Verification items for this drawing (mm, ordinates from the low corner). Coordinates: 2 decimals unless noted, no trailing zeros. Order: outer loops, then holes, each group sorted by start corner. A loop starts at its lowest first (then second) coordinate and runs counter-clockwise, first axis right, second up. Notation, with made-up numbers: M 52.5,41.5 L 69.5,41.5 A26 cw 69.5,77.5 Z; hole C 9,4 d10. An arc over 180 degrees is marked long. Return JSON: item names as keys, results as strings. Group by question number.
1. Gauge pin test, flat ends, axial feed: pin 1 (0.5 mm diameter, centred on x = 6, y = 1, fed in from -Z); pin 2 (0.8 mm diameter, centred on y = 0.5, z = 21.5, fed in from -X); pin 3 (0.8 mm diameter, centred on y = 1, z = 22.5, fed in from +X). Record the tip position at first contact, or that the pin passes through.
2. Section check A-A, the plane y = 0.3. Record the cut outline in (x, z), plus the area to 3 significant figures.
3. Section check C-C, the plane x = 24. Record the cut outline in (y, z), plus the area to 3 significant figures.
4. Material ranges on line 1 along X through (y, z) = (0.7, 9); line 2 along X through (y, z) = (0.55, 23), recorded low to high.
5. Section check B-B, the plane z = 9.5. Record the cut outline in (x, y), plus the area to 3 significant figures.
6. Section check D-D, the plane z = 20. Record the cut outline in (x, y).
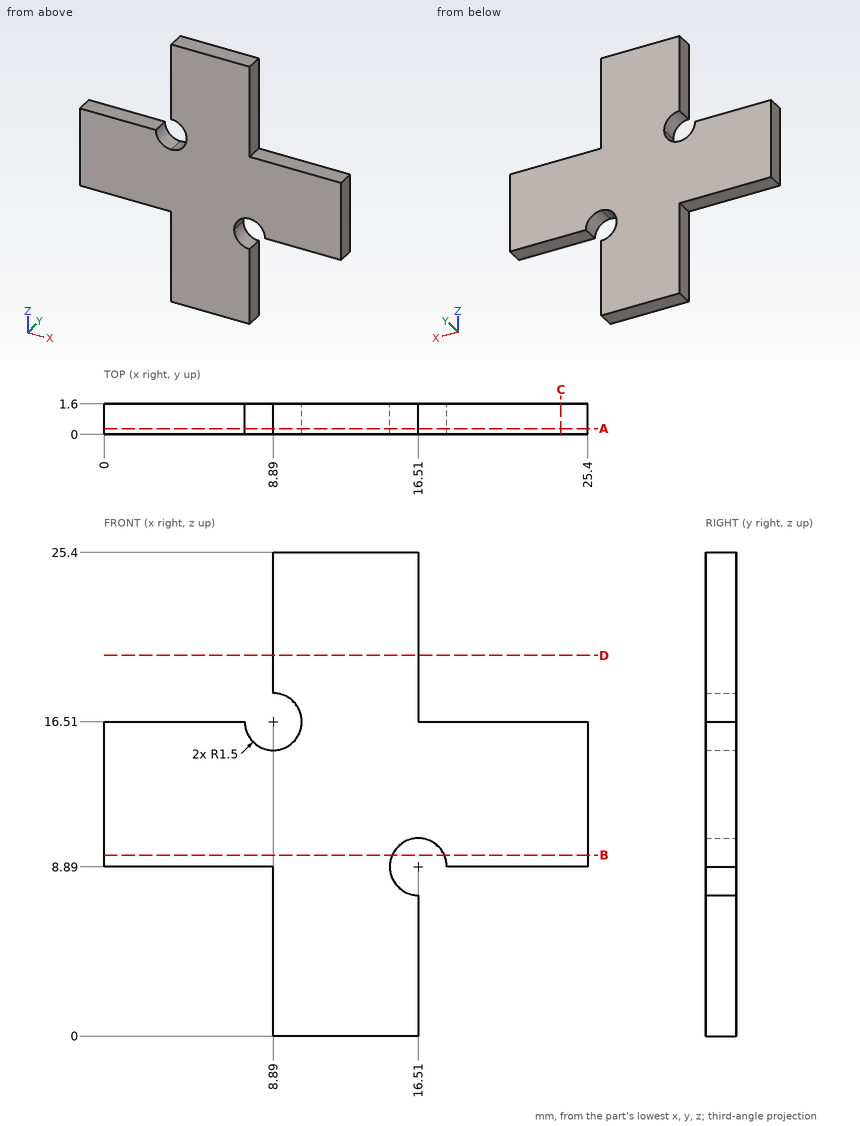
Answers follow:
{
 "1": {"pin 1": "z = 8.89", "pin 2": "x = 8.89", "pin 3": "x = 16.51"},
 "2": {"outline": "M 0,8.89 L 8.89,8.89 L 8.89,0 L 16.51,0 L 16.51,7.39 A1.5 cw long 18.01,8.89 L 25.4,8.89 L 25.4,16.51 L 16.51,16.51 L 16.51,25.4 L 8.89,25.4 L 8.89,18.01 A1.5 cw long 7.39,16.51 L 0,16.51 Z", "area": "318 mm^2"},
 "3": {"outline": "M 0,8.89 L 1.6,8.89 L 1.6,16.51 L 0,16.51 Z", "area": "12.2 mm^2"},
 "4": {"line 1": "0 to 15.01, 18.01 to 25.4", "line 2": "8.89 to 16.51"},
 "5": {"outline": "M 0,0 L 15.14,0 L 15.14,1.6 L 0,1.6 Z; M 17.88,0 L 25.4,0 L 25.4,1.6 L 17.88,1.6 Z", "area": "36.3 mm^2"},
 "6": {"outline": "M 8.89,0 L 16.51,0 L 16.51,1.6 L 8.89,1.6 Z"}
}
